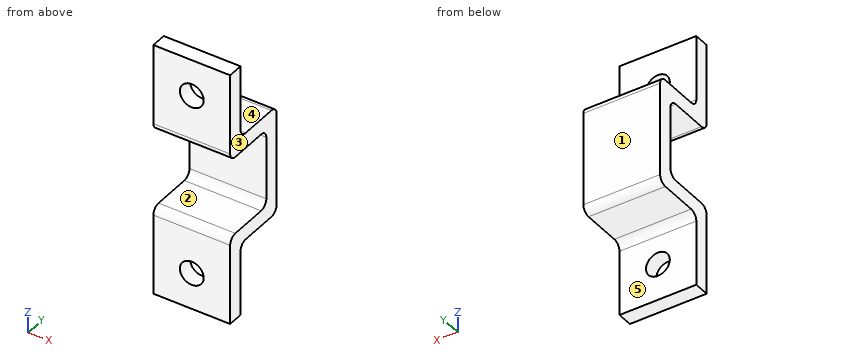
from build123d import *

# Parameters (mm, degrees)
BOSS_EXTRUDE1_DEPTH = 20
SKETCH2_R           = 3.1
CUT_EXTRUDE1_DEPTH  = 4
FILLET1_R           = 2


with BuildPart() as part:
    # Sketch1 → Boss-Extrude1 (new body)
    with BuildSketch(Plane(origin=(0, 0, 0), x_dir=(0, 0, -1), z_dir=(1, 0, 0))):
        Polygon((-10.2, 0), (10.2, 0), (10.2, -14), (33.2, -14), (33.2, -10), (14.2, -10), (14.2, 4), (-14.2, 4), (-14.2, -10), (-33.2, -10), (-33.2, -14), (-10.2, -14), align=None)
    extrude(amount=BOSS_EXTRUDE1_DEPTH)

    # Sketch2 → Cut-Extrude1 (cut)
    with BuildSketch(Plane(origin=(0, -10, 0), x_dir=(1, 0, 0), z_dir=(0, 1, 0))):
        with Locations(Location((10, 23.7, 0), (0, 0, 270))):
            Circle(SKETCH2_R)
    cut_extrude1 = extrude(amount=-CUT_EXTRUDE1_DEPTH, mode=Mode.SUBTRACT)

    # Mirror1: Cut-Extrude1 across plane
    add(cut_extrude1.mirror(Plane.XY), mode=Mode.SUBTRACT)

    # Fillet1
    fillet1_edges = [part.edges().sort_by_distance(p)[0] for p in [
        (10, -14, 10.2),
        (10, -10, 14.2),
        (10, 4, 14.2),
        (10, 4, -14.2),
        (10, -10, -14.2),
        (10, -14, -10.2),
        (10, 0, -10.2),
        (10, 0, 10.2),
    ]]
    fillet(fillet1_edges, radius=FILLET1_R)


solid = part.part
Build history of the part. All positions in model axes, mm. Face numbers are marked on the shaded views. A direction names the side the tool comes from. Coordinates: 2 decimals unless noted, no trailing zeros. Write each loop counter-clockwise with the first axis right and the second up, starting at its lowest first coordinate (ties: lowest second). Pieces come first, ordered by that corner, then holes. Notation, with made-up numbers: (18, 47) -> (74, 47) arc R33 cw to (74, 82) -> close; hole circle Ø9 at (58.5, -32). An arc over 180 degrees is marked (long way). Use CSV: the item, a comma, the result in double quotes. Start each with the question number.
Q1. Flat gauge pins, fed straight in: pin 1 Ø5 at (x, z) = (11.5, -23) entering from +Y; pin 2 Ø8 at (x, y) = (5.5, -1.5) entering from +Z; pin 3 Ø8 at (x, z) = (13, 2.5) entering from -Y; pin 4 Ø3.5 at (x, z) = (10, 23.7) entering from -Y. Where does each tip first touch, or does it go through?
Q2. 3-axis set-ups, long thin cutter, end or side, ignore diameter. For the marked faces 1, 2, 3, 4 and 5: which of +Z, -Z, +X, -X, +Y, -Y reach the whole face in a straight line?
Q3. Cut at D-D, the plane x = 10. List the corners of the cut face in (y, z).
Q4. Cut at B-B, the plane x = 5. List the corners of the cut face in (y, z).
Q5. Cut at A-A, the plane z = -23.7. List the corners of the cut face in (x, y).
Q6. Cut at C-C, the plane y = -7.25. List the corners of the cut face in (x, z), then the cut area to 3 significant figures.
Q7. Drill centre lines: probe 1 along X at (y, z) = (-11.8, -23.7); probe 2 along Z at (x, y) = (15.5, -5); probe 3 along Y at (x, z) = (4, -4.5). Where is each one in solid material? Low to high.
Checked values:
1,pin 1,"stops at y = -10"
1,pin 2,"stops at z = 14.2"
1,pin 3,"stops at y = 0"
1,pin 4,"passes through"
2,face 1,"+Z, -Z, +X, -X, +Y"
2,face 2,"+X, -X, -Y"
2,face 3,"+Z, -Z, +X, +Y, -Y"
2,face 4,"+Z, +X, -X, +Y"
2,face 5,"-Z, +X, -X, +Y"
3,outline,"(-14, -33.2) -> (-10, -33.2) -> (-10, -26.8) -> (-14, -26.8) -> close; (-14, -20.6) -> (-10, -20.6) -> (-10, -16.2) arc R2 cw to (-8, -14.2) -> (2, -14.2) arc R2 ccw to (4, -12.2) -> (4, 12.2) arc R2 ccw to (2, 14.2) -> (-8, 14.2) arc R2 cw to (-10, 16.2) -> (-10, 20.6) -> (-14, 20.6) -> (-14, 12.2) arc R2 ccw to (-12, 10.2) -> (-2, 10.2) arc R2 cw to (0, 8.2) -> (0, -8.2) arc R2 cw to (-2, -10.2) -> (-12, -10.2) arc R2 ccw to (-14, -12.2) -> close; (-14, 26.8) -> (-10, 26.8) -> (-10, 33.2) -> (-14, 33.2) -> close"
4,outline,"(-14, -33.2) -> (-10, -33.2) -> (-10, -16.2) arc R2 cw to (-8, -14.2) -> (2, -14.2) arc R2 ccw to (4, -12.2) -> (4, 12.2) arc R2 ccw to (2, 14.2) -> (-8, 14.2) arc R2 cw to (-10, 16.2) -> (-10, 33.2) -> (-14, 33.2) -> (-14, 12.2) arc R2 ccw to (-12, 10.2) -> (-2, 10.2) arc R2 cw to (0, 8.2) -> (0, -8.2) arc R2 cw to (-2, -10.2) -> (-12, -10.2) arc R2 ccw to (-14, -12.2) -> close"
5,outline,"(0, -14) -> (6.9, -14) -> (6.9, -10) -> (0, -10) -> close; (13.1, -14) -> (20, -14) -> (20, -10) -> (13.1, -10) -> close"
6,outline,"(0, -14.2) -> (20, -14.2) -> (20, -10.2) -> (0, -10.2) -> close; (0, 10.2) -> (20, 10.2) -> (20, 14.2) -> (0, 14.2) -> close"
6,area,"160 mm²"
7,probe 1,"x = 0 to 6.9, 13.1 to 20"
7,probe 2,"z = -14.2 to -10.2, 10.2 to 14.2"
7,probe 3,"y = 0 to 4"
